```python
from build123d import *

# Parameters (mm, degrees)
SKETCH1_R                            = 43
SKETCH1_R_2                          = 40
BOSS_EXTRUDE1_DEPTH                  = 63
SKETCH2_R                            = 41.5
SKETCH2_R_2                          = 40
CUT_EXTRUDE1_DEPTH                   = 3
BOSS_EXTRUDE2_REACH                  = 89.561
BOSS_EXTRUDE2_END_RADIUS             = 40
BOSS_EXTRUDE2_DIRECTION_2_REACH      = 89.561
BOSS_EXTRUDE2_DIRECTION_2_END_RADIUS = 40
BOSS_EXTRUDE3_DEPTH                  = 70
CUT_EXTRUDE2_REACH                   = 125.284
CUT_EXTRUDE2_END_RADIUS              = 40
CUT_EXTRUDE3_DEPTH                   = 100.163089401
BOSS_EXTRUDE6_DEPTH                  = 3
CUT_EXTRUDE4_DEPTH                   = 4


with BuildPart() as part:
    # Sketch1 → Boss-Extrude1 (new body)
    with BuildSketch(Plane(origin=(0, 0, 0), x_dir=(1, 0, 0), z_dir=(0, 1, 0))):
        with Locations(Location((0, 0, 0), (0, 0, 270))):
            Circle(SKETCH1_R)
        with Locations(Location((0, 0, 0), (0, 0, 270))):
            Circle(SKETCH1_R_2, mode=Mode.SUBTRACT)
    extrude(amount=BOSS_EXTRUDE1_DEPTH)

    # Sketch2 → Cut-Extrude1 (cut)
    with BuildSketch(Plane(origin=(0, 0, 0), x_dir=(-1, 0, 0), z_dir=(0, -1, 0))):
        with Locations(Location((0, 0, 0), (0, 0, 90))):
            Circle(SKETCH2_R)
        with Locations(Location((0, 0, 0), (0, 0, 90))):
            Circle(SKETCH2_R_2, mode=Mode.SUBTRACT)
    extrude(amount=-CUT_EXTRUDE1_DEPTH, mode=Mode.SUBTRACT)

    # Boss-Extrude2: up to this cylinder (the profile starts inside it)
    boss_extrude2_end = Plane(origin=(0, 21.31795, 0), z_dir=(0, -1, 0)) * Cylinder(BOSS_EXTRUDE2_END_RADIUS, 260.122, mode=Mode.PRIVATE)
    # Sketch4 → Boss-Extrude2 (add, up to the surface)
    with BuildSketch(Plane(origin=(0, 0, 0), x_dir=(0, 0, -1), z_dir=(1, 0, 0)), mode=Mode.PRIVATE) as boss_extrude2_sk1:
        Polygon((-23, 13), (43, 30.6846467), (43, 28.541053161), (-15, 13), align=None)
    boss_extrude2_tool1 = extrude(boss_extrude2_sk1.sketch, amount=-BOSS_EXTRUDE2_REACH, mode=Mode.PRIVATE) & boss_extrude2_end
    add(boss_extrude2_tool1.solids().sort_by_distance((0, 21.31795, -11.956989))[0])

    # Boss-Extrude2 direction 2: up to this cylinder (the profile starts inside it)
    boss_extrude2_direction_2_end = Plane(origin=(0, 21.31795, 0), z_dir=(0, -1, 0)) * Cylinder(BOSS_EXTRUDE2_DIRECTION_2_END_RADIUS, 260.122, mode=Mode.PRIVATE)
    # Sketch4 → Boss-Extrude2 direction 2 (add, up to the surface)
    with BuildSketch(Plane(origin=(0, 0, 0), x_dir=(0, 0, -1), z_dir=(1, 0, 0)), mode=Mode.PRIVATE) as boss_extrude2_direction_2_sk1:
        Polygon((-23, 13), (43, 30.6846467), (43, 28.541053161), (-15, 13), align=None)
    boss_extrude2_direction_2_tool1 = extrude(boss_extrude2_direction_2_sk1.sketch, amount=BOSS_EXTRUDE2_DIRECTION_2_REACH, mode=Mode.PRIVATE) & boss_extrude2_direction_2_end
    add(boss_extrude2_direction_2_tool1.solids().sort_by_distance((0, 21.31795, -11.956989))[0])


with BuildPart() as body_2:
    # Sketch5 → Boss-Extrude3 (new body)
    with BuildSketch(Plane(origin=(0, 63, 0), x_dir=(1, 0, 0), z_dir=(0, 1, 0))):
        Polygon((7.74910462, -54.037683176), (34.954425762, -25.676995378), (36.517040035, -27.175951378), (9.311718893, -55.536639176), align=None)
    extrude(amount=-BOSS_EXTRUDE3_DEPTH)


with BuildPart() as cut_extrude2_tool:
    # Cut-Extrude2: up to this cylinder (the profile starts outside it)
    cut_extrude2_end = Plane(origin=(0, 7.120173, 0), z_dir=(0, -1, 0)) * Cylinder(CUT_EXTRUDE2_END_RADIUS, 331.568, mode=Mode.PRIVATE)
    # Sketch6 → Cut-Extrude2 (new, up to the surface)
    with BuildSketch(Plane(origin=(32.59371092, 0, 31.265898031), x_dir=(0.6922545038449902, 0, -0.7216534500065296), z_dir=(0.7216534500065296, 0, 0.6922545038449902)), mode=Mode.PRIVATE) as cut_extrude2_sk1:
        with BuildLine():
            Line((-18.432533638, 7.25), (-18.432533638, 3))
            Line((-18.432533638, 3), (5.667466362, 3))
            Line((5.667466362, 3), (5.667466362, 7.25))
            ThreePointArc((5.667466362, 7.25), (4.422670182, 10.25520382), (1.417466362, 11.5))
            Line((1.417466362, 11.5), (-14.182533638, 11.5))
            ThreePointArc((-14.182533638, 11.5), (-17.187737458, 10.25520382), (-18.432533638, 7.25))
        make_face()
    cut_extrude2_tool1 = extrude(cut_extrude2_sk1.sketch, amount=-CUT_EXTRUDE2_REACH, mode=Mode.PRIVATE) - cut_extrude2_end
    add(cut_extrude2_tool1.solids().sort_by_distance((28.175373, 7.120173, 35.871875))[0])


with BuildPart() as part_1:
    add(part.part)

    # Cut-Extrude2: cut by cut_extrude2_tool
    add(cut_extrude2_tool.part, mode=Mode.SUBTRACT)

    # Sketch11 → Boss-Extrude6 (add)
    with BuildSketch(Plane(origin=(0, 3, 0), x_dir=(1, 0, 0), z_dir=(0, 1, 0))):
        Polygon((14.90592475, -39.87722305), (34.683715998, -25.417313874), (48.112422428, -42.207782707), (26.881207412, -57.733387396), align=None)
    extrude(amount=-BOSS_EXTRUDE6_DEPTH)

    # Sketch12 → Cut-Extrude4 (cut)
    with BuildSketch(Plane(origin=(0, 0, 0), x_dir=(-1, 0, 0), z_dir=(0, -1, 0))):
        with BuildLine():
            Line((-30.912368333, -27.688857915), (-14.530563251, -38.873033476))
            ThreePointArc((-14.530563251, -38.873033476), (-23.375174905, -34.238453489), (-30.912368333, -27.688857915))
        make_face()
    extrude(amount=-CUT_EXTRUDE4_DEPTH, mode=Mode.SUBTRACT)


with BuildPart() as body_2_1:
    add(body_2.part)

    # Cut-Extrude2: cut by cut_extrude2_tool
    add(cut_extrude2_tool.part, mode=Mode.SUBTRACT)

    # Sketch7 → Cut-Extrude3 (cut, through all)
    with BuildSketch(Plane(origin=(0, 63, 0), x_dir=(1, 0, 0), z_dir=(0, 1, 0))):
        Polygon((34.954425762, -25.676995378), (36.517040035, -27.175951378), (9.311718893, -55.536639176), (7.74910462, -54.037683176), align=None)
    extrude(amount=-CUT_EXTRUDE3_DEPTH, mode=Mode.SUBTRACT)


solid = part_1.part
```
Geometry check sheet. Reference: the model listing, model coordinates, mm. A direction names the side the tool comes from. Coordinates: 2 decimals unless noted, no trailing zeros. Order: outer loops, then holes, each group sorted by start corner. A loop starts at its lowest first (then second) coordinate and runs counter-clockwise, first axis right, second up.
Item 1: Scan lines: line 1 along X through (y, z) = (29, 0); line 2 along Z through (x, y) = (0, 0.9). Record each from-to range of solid material in increasing order.
Item 2: Section check D-D (y = 35). Enter the section's corners in (x, z).
Item 3: Section check C-C (x = 25.5). Enter the section's corners in (y, z).
Item 4: Section check A-A (x = 0). Enter the section's corners in (y, z).
Item 5: Section check B-B (z = 17). Enter the section's corners in (x, y), plus the area to 3 significant figures.
Item 6: Tool access check on faces 5 (the flat face through (-1, 13, 19)), 6 (the cylindrical face through (15.61, 10.29, 38.74)), 7 (the flat face through (-38, 63, 13)), 8 (the cylindrical face through (-15.32, 32.58, 36.95)), 9 (the flat face through (41.304, 1.521, 33.695)). Record the directions out of +Z, -Z, +X, -X, +Y, -Y that give a thin tool (end or side, any length) a straight path to the whole face; none if there is none.
Item 7: Mould release check, pull along Y, two halves, no side actions. Record for faces 1 (the flat face through (14.08, 5.15, 39.05)), 2 (the flat face through (-0.56, 21.322, -8.059)), 3 (the flat face through (21.1, 1.52, 49.11)), 4 (the cylindrical face through (32.9, 10.22, 25.38)): released by +Y, released by -Y, zero draft, split by the parting line, or undercut.
Item 8: Depth check by flat-ended pin: pin 1 (3 mm diameter, centred on x = 28, y = 51, fed in from -Z); pin 2 (3 mm diameter, centred on x = 30.5, y = 30, fed in from +Z); pin 3 (10 mm diameter, centred on x = 23, z = 49.5, fed in from +Y); pin 4 (9.5 mm diameter, centred on x = 24, z = 31.5, fed in from -Y). Enter the tip coordinate at first touch or a pass-through.
Check sheet entries:
1. line 1: x = -43 to -40, 40 to 43
1. line 2: z = -43 to -41.5, 41.5 to 43
2. outline: circle Ø86 at (0, 0); hole circle Ø80 at (0, 0)
3. outline: (0, -34.62) - (63, -34.62) - (63, -30.82) - (27.42, -30.82) - (13, 23) - (13, 15) - (25.28, -30.82) - (3, -30.82) - (3, -32.74) - (0, -32.74) - close; (0, 32.69) - (3, 32.69) - (3, 55.67) - (0, 55.67) - close; (11.5, 30.82) - (63, 30.82) - (63, 34.62) - (11.5, 34.62) - close
4. outline: (0, -43) - (63, -43) - (63, -40) - (29.88, -40) - (13, 23) - (13, 15) - (27.74, -40) - (3, -40) - (3, -41.5) - (0, -41.5) - close; (0, 41.5) - (3, 41.5) - (3, 40) - (63, 40) - (63, 43) - (0, 43) - close
5. outline: (-39.5, 0) - (-37.86, 0) - (-37.86, 3) - (-36.21, 3) - (-36.21, 13) - (36.21, 13) - (36.21, 3) - (37.86, 3) - (37.86, 0) - (39.5, 0) - (39.5, 63) - (36.21, 63) - (36.21, 14.61) - (-36.21, 14.61) - (-36.21, 63) - (-39.5, 63) - close
5. area: 521 mm2
6. face 5: -Y
6. face 6: +X
6. face 7: +Z, -Z, +X, -X, +Y
6. face 8: none
6. face 9: +X, +Y, -Y
7. face 1: undercut
7. face 2: released by +Y
7. face 3: zero draft
7. face 4: undercut
8. pin 1: stops at z = -33.86
8. pin 2: stops at z = 31.75
8. pin 3: stops at y = 3
8. pin 4: stops at y = 0
